For this review, take the finished solid that the model builds, in its own axes (mm). A direction names the side the tool comes from. Round coordinates to 2 decimals unless told otherwise and drop trailing zeros. Loops run counter-clockwise (first coordinate to the right, second up) from the corner with the lowest first, then second, coordinate; pieces in that order, holes last. Notation, with made-up numbers: M 5,9 L 21,9 A35 ccw 21,48 Z; hole C -28,-28.75 d1. An arc over 180 degrees is marked long. One line per question, with ' | ' between items. Start each with the question number.
1) For faces 4 (the face through (34.886, -13.739, -1.711)), 5 (the face through (13.1, -13.7, 1.2)), 6 (the face through (7.97, -4.78, 3.71)), list the 3-axis set-ups (+Z, -Z, +X, -X, +Y, -Y) from which the entire face can be reached by the end or side of a thin tool; tool diameter is ignored.
2) We need section C-C (z = 0.75). State how many separate pieces and enclosed holes the cut face has, and give its area (3 significant figures).
3) For pin 1 Ø2 at (x, y) = (12.5, 1.5) entering from -Z; pin 2 Ø5 at (x, y) = (-8, -10.5) entering from -Z; pin 3 Ø0.6 at (y, z) = (-16.5, 1.5) entering from -X, all flat-tipped, find the tip position at first contact; note any pin that passes through.
4) For probe 1 along Y at (x, z) = (-13.1, 3.25) (3 decimals); probe 2 along X at (y, z) = (-1, 1); probe 3 along Z at (x, y) = (3, -16.25), list the stretches that pass through material, from the lowest coordinate up. Write a range as from..to.
5) We need section D-D (x = 7.5). Give the boundary of the cut face in (y, z) (3 decimals), and give its area (3 significant figures).
6) We need section B-B (x = -4.5). Give the boundary of the cut face in (y, z), and give its area (3 significant figures).
7) We need section A-A (x = -13.1). Give the boundary of the cut face in (y, z) (3 decimals), and give its area (3 significant figures).
8) Mouldability with a two-part tool opening along X and no side actions: class faces 1 (the face through (-6.3, -6, 3)), 2 (the face through (-38.57, -3.85, -16.19)), 3 (the face through (-23, -0.96, 3)) as pulls with the +X half, pulls with the -X half, needs draft (parallel to the pull), parting line crosses it, or undercut.
```python
from build123d import *

# Parameters (mm, degrees)
SKETCH_1_W                   = 135
SKETCH_1_H                   = 58
EXTRUDE_1_DEPTH              = 10
SKETCH_3_W                   = 20.3
SKETCH_3_H                   = 40.5
CUT_EXTRUDE_1_DEPTH          = 20
SKETCH_4_R                   = 1.525
CUT_EXTRUDE_2_DEPTH          = 20
SKETCH_5_W                   = 45
SKETCH_5_H                   = 15.3
CUT_EXTRUDE_3_DEPTH          = 20
SKETCH_7_R                   = 2.575
CUT_EXTRUDE_4_DEPTH          = 57
SKETCH_9_W                   = 49.35
SKETCH_9_H                   = 22.8
CUT_EXTRUDE_6_DEPTH          = 48
FILLET_1_R                   = 3
FILLET_2_R                   = 3
CUT_EXTRUDE_START            = -57
SKETCH_10_R                  = 2.575
CUT_EXTRUDE_7_DEPTH          = 57
EXTRUDE_2_DEPTH              = 28
SKETCH_12_R                  = 2.575
CUT_EXTRUDE_8_DEPTH          = 145
CUT_EXTRUDE_9_DEPTH          = 145
FILLET_3_R                   = 6
FILLET_4_R                   = 10
SKETCH_14_R                  = 1
CUT_EXTRUDE_10_DEPTH         = 135
SKETCH_15_W                  = 2
SKETCH_15_H                  = 13
CUT_EXTRUDE_11_DEPTH         = 1.5
EXTRUDE_3_DEPTH              = 10
SKETCH_17_R                  = 1.5
CUT_EXTRUDE_12_DEPTH         = 8
FILLET_6_R                   = 10
SKETCH_18_R                  = 1.5
CUT_EXTRUDE_13_DEPTH         = 8
CUT_EXTRUDE_START_2          = -1
CUT_EXTRUDE_14_DEPTH         = 1
CUT_EXTRUDE_15_DEPTH         = 1
SCALE_1_SCALE                = 0.6
SKETCH_21_W                  = 36.846511631
SKETCH_21_H                  = 29.09734836
CUT_EXTRUDE_16_DEPTH         = 10
DELETE_FACE_1_OUTLINE_R      = 0.915
DELETE_FACE_1_DEPTH          = 6
DELETE_START                 = 12.6
DELETE_FACE_1_2_OUTLINE_R    = 0.9
DELETE_FACE_1_2_DEPTH        = 4.8
SKETCH_22_W                  = 42.319658251
SKETCH_22_H                  = 16.876277442
CUT_EXTRUDE_17_DEPTH         = 10
SKETCH_23_W                  = 12.18
SKETCH_23_H                  = 4.68
EXTRUDE_4_DEPTH              = 6
HOLE_WIZARD_M2_1_D           = 2.4
HOLE_WIZARD_M2_1_CBORE_D     = 4.4
HOLE_WIZARD_M2_1_CBORE_DEPTH = 2.4
SKETCH_28_W                  = 4.4
SKETCH_28_H                  = 3.92528177
SKETCH_28_H_2                = 4.286505362
CUT_EXTRUDE_18_DEPTH         = 2.4


# Read off the part's stored shape, not the designer's step: 删除面1
with BuildPart() as part:
    # 草图1 → 凸台-拉伸1 (new body)
    with BuildSketch(Plane.XY):
        Rectangle(SKETCH_1_W, SKETCH_1_H)
    extrude(amount=EXTRUDE_1_DEPTH)

    # 草图3 → 切除-拉伸1 (cut)
    with BuildSketch(Plane(origin=(0, 0, 0), x_dir=(-1, 0, 0), z_dir=(0, 0, -1))):
        Rectangle(SKETCH_3_W, SKETCH_3_H)
    extrude(amount=-CUT_EXTRUDE_1_DEPTH, mode=Mode.SUBTRACT)

    # 草图4 → 切除-拉伸2 (cut)
    with BuildSketch(Plane(origin=(0, 0, 0), x_dir=(-1, 0, 0), z_dir=(0, 0, -1))):
        with Locations((-5, 24.6)):
            Circle(SKETCH_4_R)
        with Locations(Location((5, 24.6, 0), (0, 0, 180))):
            Circle(SKETCH_4_R)
        with Locations((5, -24.6)):
            Circle(SKETCH_4_R)
        with Locations(Location((-5, -24.6, 0), (0, 0, 180))):
            Circle(SKETCH_4_R)
    extrude(amount=-CUT_EXTRUDE_2_DEPTH, mode=Mode.SUBTRACT)

    # 草图5 → 切除-拉伸3 (cut)
    with BuildSketch(Plane(origin=(0, 0, 0), x_dir=(-1, 0, 0), z_dir=(0, 0, -1))):
        with Locations((38.65, -10.25)):
            Rectangle(SKETCH_5_W, SKETCH_5_H)
        with Locations((-38.65, -10.25)):
            Rectangle(SKETCH_5_W, SKETCH_5_H)
    extrude(amount=-CUT_EXTRUDE_3_DEPTH, mode=Mode.SUBTRACT)

    # 草图7 → 切除-拉伸4 (cut)
    with BuildSketch(Plane.ZY.offset(67.5)):
        with Locations((5, -10.25)):
            Circle(SKETCH_7_R)
    extrude(amount=-CUT_EXTRUDE_4_DEPTH, mode=Mode.SUBTRACT)

    # 草图9 → 切除-拉伸6 (cut)
    with BuildSketch(Plane(origin=(0, 0, 0), x_dir=(-1, 0, 0), z_dir=(0, 0, -1))):
        with Locations((-42.825, 17.6)):
            Rectangle(SKETCH_9_W, SKETCH_9_H)
        with Locations((42.825, 17.6)):
            Rectangle(SKETCH_9_W, SKETCH_9_H)
    extrude(amount=-CUT_EXTRUDE_6_DEPTH, mode=Mode.SUBTRACT)

    # 圆角1
    fillet_1_edges = [part.edges().sort_by_distance(p)[0] for p in [
        (18.15, 29, 5),
        (18.15, 6.2, 5),
        (-18.15, 29, 5),
        (-18.15, 6.2, 5),
    ]]
    fillet(fillet_1_edges, radius=FILLET_1_R)

    # 圆角2
    fillet_2_edges = [part.edges().sort_by_distance(p)[0] for p in [
        (67.5, 6.2, 5),
        (-67.5, 6.2, 5),
        (67.5, -29, 5),
        (-67.5, -29, 5),
    ]]
    fillet(fillet_2_edges, radius=FILLET_2_R)

    # 草图10 → 切除-拉伸7 (cut)
    with BuildSketch(Plane(origin=(67.5, 0, 0), x_dir=(0, 0, -1), z_dir=(1, 0, 0)).offset(CUT_EXTRUDE_START)):
        with Locations(Location((-5, -10.25, 0), (0, 0, 180))):
            Circle(SKETCH_10_R)
    extrude(amount=CUT_EXTRUDE_7_DEPTH, mode=Mode.SUBTRACT)

    # 草图11 → 凸台-拉伸2 (add)
    with BuildSketch(Plane(origin=(0, 0, 0), x_dir=(-1, 0, 0), z_dir=(0, 0, -1))):
        with BuildLine():
            Line((61.15, 6.2), (61.15, -29))
            Line((61.15, -29), (64.5, -29))
            ThreePointArc((64.5, -29), (66.621320344, -28.121320344), (67.5, -26))
            Line((67.5, -26), (67.5, 3.2))
            ThreePointArc((67.5, 3.2), (66.621320344, 5.321320344), (64.5, 6.2))
            Line((64.5, 6.2), (61.15, 6.2))
        make_face()
        with BuildLine():
            Line((-61.15, 6.2), (-61.15, -29))
            Line((-61.15, -29), (-64.5, -29))
            ThreePointArc((-64.5, -29), (-66.621320344, -28.121320344), (-67.5, -26))
            Line((-67.5, -26), (-67.5, 3.2))
            ThreePointArc((-67.5, 3.2), (-66.621320344, 5.321320344), (-64.5, 6.2))
            Line((-64.5, 6.2), (-61.15, 6.2))
        make_face()
    extrude(amount=EXTRUDE_2_DEPTH)

    # 草图12 → 切除-拉伸8 (cut)
    with BuildSketch(Plane.ZY.offset(67.5)):
        with Locations((-21, -10.25)):
            Circle(SKETCH_12_R)
    extrude(amount=-CUT_EXTRUDE_8_DEPTH, mode=Mode.SUBTRACT)

    # 草图13 → 切除-拉伸9 (cut)
    with BuildSketch(Plane.ZY.offset(67.5)):
        Polygon((-28, 6.2), (-28, -5.8), (0, 6.2), align=None)
        Polygon((0, -29), (-28, -29), (-28, -17), align=None)
    extrude(amount=-CUT_EXTRUDE_9_DEPTH, mode=Mode.SUBTRACT)

    # 圆角3
    fillet_3_edges = [part.edges().sort_by_distance(p)[0] for p in [
        (64.325, -17, -28),
        (64.325, -5.8, -28),
        (-64.325, -5.8, -28),
        (-64.325, -17, -28),
    ]]
    fillet(fillet_3_edges, radius=FILLET_3_R)

    # 圆角4
    fillet_4_edges = [part.edges().sort_by_distance(p)[0] for p in [
        (-61.15, 1.8, 0),
        (-61.15, -23.45, 0),
        (61.15, -23.45, 0),
        (61.15, 1.8, 0),
    ]]
    fillet(fillet_4_edges, radius=FILLET_4_R)

    # 草图14 → 切除-拉伸10 (cut)
    with BuildSketch(Plane.ZY.offset(67.5)):
        with Locations((-13, -10.25)):
            Circle(SKETCH_14_R)
        with Locations((-3, -10.25)):
            Circle(SKETCH_14_R)
    extrude(amount=-CUT_EXTRUDE_10_DEPTH, mode=Mode.SUBTRACT)

    # 草图15 → 切除-拉伸11 (cut)
    with BuildSketch(Plane.XY.offset(10)):
        with Locations((0, 20.25)):
            Rectangle(SKETCH_15_W, SKETCH_15_H)
        with Locations((0, -20.25)):
            Rectangle(SKETCH_15_W, SKETCH_15_H)
    extrude(amount=-CUT_EXTRUDE_11_DEPTH, mode=Mode.SUBTRACT)

    # 草图16 → 凸台-拉伸3 (add)
    with BuildSketch(Plane(origin=(0, 0, 0), x_dir=(-1, 0, 0), z_dir=(0, 0, -1))):
        with BuildLine():
            Line((-18.15, 20.25), (18.15, 20.25))
            Line((18.15, 20.25), (18.15, 26))
            ThreePointArc((18.15, 26), (17.271320344, 28.121320344), (15.15, 29))
            Line((15.15, 29), (-15.15, 29))
            ThreePointArc((-15.15, 29), (-17.271320344, 28.121320344), (-18.15, 26))
            Line((-18.15, 26), (-18.15, 20.25))
        make_face()
    extrude(amount=EXTRUDE_3_DEPTH)

    # 草图17 → 切除-拉伸12 (cut)
    with BuildSketch(Plane(origin=(0, 29, 0), x_dir=(1, 0, 0), z_dir=(0, 1, 0))):
        with Locations(Location((-9, 6, 0), (0, 0, 270))):
            Circle(SKETCH_17_R)
        with Locations(Location((9, 6, 0), (0, 0, 270))):
            Circle(SKETCH_17_R)
        with Locations(Location((9, -6, 0), (0, 0, 270))):
            Circle(SKETCH_17_R)
        with Locations(Location((-9, -6, 0), (0, 0, 270))):
            Circle(SKETCH_17_R)
    extrude(amount=-CUT_EXTRUDE_12_DEPTH, mode=Mode.SUBTRACT)

    # 圆角6
    fillet_6_edges = [part.edges().sort_by_distance(p)[0] for p in [
        (-14.15, 20.25, 0),
        (14.15, 20.25, 0),
    ]]
    fillet(fillet_6_edges, radius=FILLET_6_R - 0.0001)  # a hair under: the kernel refuses the full size

    # 草图18 → 切除-拉伸13 (cut)
    with BuildSketch(Plane(origin=(0, 21, 0), x_dir=(1, 0, 0), z_dir=(0, 1, 0))):
        with Locations(Location((9, 6, 0), (0, 0, 270))):
            Circle(SKETCH_18_R)
        with Locations(Location((-9, 6, 0), (0, 0, 270))):
            Circle(SKETCH_18_R)
    extrude(amount=-CUT_EXTRUDE_13_DEPTH, mode=Mode.SUBTRACT)

    # 草图19 → 切除-拉伸14 (cut)
    with BuildSketch(Plane(origin=(0, -17.9, 0), x_dir=(1, 0, 0), z_dir=(0, 1, 0)).offset(CUT_EXTRUDE_START_2)):
        with BuildLine():
            Line((16.15, -10), (61.15, -10))
            Line((61.15, -10), (61.15, 10))
            ThreePointArc((61.15, 10), (58.221067812, 2.928932188), (51.15, 0))
            Line((51.15, 0), (16.15, 0))
            Line((16.15, 0), (16.15, -10))
        make_face()
        with BuildLine():
            Line((-61.15, -10), (-16.15, -10))
            Line((-16.15, -10), (-16.15, 0))
            Line((-16.15, 0), (-51.15, 0))
            ThreePointArc((-51.15, 0), (-58.221067812, 2.928932188), (-61.15, 10))
            Line((-61.15, 10), (-61.15, -10))
        make_face()
    extrude(amount=CUT_EXTRUDE_14_DEPTH, mode=Mode.SUBTRACT)

    # 草图20 → 切除-拉伸15 (cut)
    with BuildSketch(Plane.XZ.offset(2.6)):
        with BuildLine():
            Line((-16.15, 10), (-61.15, 10))
            Line((-61.15, 10), (-61.15, -10))
            ThreePointArc((-61.15, -10), (-58.221067812, -2.928932188), (-51.15, 0))
            Line((-51.15, 0), (-16.15, 0))
            Line((-16.15, 0), (-16.15, 10))
        make_face()
        with BuildLine():
            Line((61.15, 10), (16.15, 10))
            Line((16.15, 10), (16.15, 0))
            Line((16.15, 0), (51.15, 0))
            ThreePointArc((51.15, 0), (58.221067812, -2.928932188), (61.15, -10))
            Line((61.15, -10), (61.15, 10))
        make_face()
    extrude(amount=-CUT_EXTRUDE_15_DEPTH, mode=Mode.SUBTRACT)


with BuildPart() as part_1:
    # 缩放比例1: scaled about (0, 0, 0)
    add(part.part.scale(SCALE_1_SCALE))

    # 草图21 → 切除-拉伸16 (cut)
    with BuildSketch(Plane(origin=(0, 0, 0), x_dir=(-1, 0, 0), z_dir=(0, 0, -1))):
        with Locations((0.657510419, 15.53719691)):
            Rectangle(SKETCH_21_W, SKETCH_21_H)
    extrude(amount=CUT_EXTRUDE_16_DEPTH, mode=Mode.SUBTRACT)

    # Delete Face 1 outline → Delete Face 1 (add)
    with BuildSketch(Plane.XY):
        with Locations((3, 14.76)):
            Circle(DELETE_FACE_1_OUTLINE_R)
        with Locations((-3, 14.76)):
            Circle(DELETE_FACE_1_OUTLINE_R)
        with Locations((-3, -14.76)):
            Circle(DELETE_FACE_1_OUTLINE_R)
        with Locations((3, -14.76)):
            Circle(DELETE_FACE_1_OUTLINE_R)
    extrude(amount=DELETE_FACE_1_DEPTH)

    # Delete Face 1 2 outline → Delete Face 1 2 (add)
    with BuildSketch(Plane(origin=(0, 0, 0), x_dir=(1, 0, 0), z_dir=(0, 1, 0)).offset(DELETE_START)):
        with Locations((5.4, -3.6)):
            Circle(DELETE_FACE_1_2_OUTLINE_R)
        with Locations((-5.4, -3.6)):
            Circle(DELETE_FACE_1_2_OUTLINE_R)
    extrude(amount=DELETE_FACE_1_2_DEPTH)

    # 草图22 → 切除-拉伸17 (cut)
    with BuildSketch(Plane(origin=(0, 0, 0), x_dir=(-1, 0, 0), z_dir=(0, 0, -1))):
        with Locations((1.658514494, 12.158138721)):
            Rectangle(SKETCH_22_W, SKETCH_22_H)
    extrude(amount=-CUT_EXTRUDE_17_DEPTH, mode=Mode.SUBTRACT)

    # 草图23 → 凸台-拉伸4 (add)
    with BuildSketch(Plane(origin=(0, 0, 0), x_dir=(-1, 0, 0), z_dir=(0, 0, -1))):
        with Locations((0, 1.38)):
            Rectangle(SKETCH_23_W, SKETCH_23_H)
    extrude(amount=-EXTRUDE_4_DEPTH)

    # M2 六角凹头螺钉的柱形沉头孔1 (through all)
    with Locations(Plane(origin=(0, 0, 0), x_dir=(-1, 0, 0), z_dir=(0, 0, -1))):
        with Locations((13.1, 1.355), (-13.1, 1.355), (-13.1, -15.9), (13.1, -15.538776408)):
            CounterBoreHole(HOLE_WIZARD_M2_1_D / 2, HOLE_WIZARD_M2_1_CBORE_D / 2, HOLE_WIZARD_M2_1_CBORE_DEPTH)

    # 草图28 → 切除-拉伸18 (cut)
    with BuildSketch(Plane(origin=(0, 0, 0), x_dir=(-1, 0, 0), z_dir=(0, 0, -1))):
        with Locations((-13.1, -17.862640885)):
            Rectangle(SKETCH_28_W, SKETCH_28_H)
        with Locations((13.1, -17.682029089)):
            Rectangle(SKETCH_28_W, SKETCH_28_H_2)
    extrude(amount=-CUT_EXTRUDE_18_DEPTH, mode=Mode.SUBTRACT)


solid = part_1.part
```
Answers below:
1) face 4: -Z, +Y, -Y | face 5: -Z, -Y | face 6: +X
2) separate pieces: 1 | enclosed holes: 5 | area: 951 mm^2
3) pin 1: z = 2.4 | pin 2: z = 0 | pin 3: x = -40.4
4) probe 1: -17.4..-16.739, -14.339..-11.34, -0.96..0.155, 2.555..3.72 | probe 2: -40.5..-36.69, -9.69..-6.09, 6.09..9.69, 36.69..40.5 | probe 3: 0..6
5) outline: M -17.4,0 L 3.72,0 L 3.72,6 L -17.4,6 Z; hole C -6.15,3 d3.09 | area: 119 mm^2
6) outline: M -17.4,0 L -12.15,0 L -12.15,6 L -17.4,6 Z; M -0.96,0 L 3.72,0 L 3.72,6 L -0.96,6 Z | area: 59.6 mm^2
7) outline: M -17.4,2.4 L -16.739,2.4 L -16.739,6 L -17.4,6 Z; M -14.339,2.4 L -13.339,2.4 L -13.339,0 L -11.34,0 L -11.34,6 L -14.339,6 Z; M -0.96,0 L -0.845,0 L -0.845,2.4 L 0.155,2.4 L 0.155,6 L -0.96,6 Z; M 2.555,2.4 L 3.555,2.4 L 3.555,0 L 3.72,0 L 3.72,6 L 2.555,6 Z | area: 26.9 mm^2
8) face 1: pulls with the -X half | face 2: needs draft | face 3: undercut
